from build123d import *

# Parameters (mm, degrees)
SKETCH1_R           = 2.4
BOSS_EXTRUDE1_DEPTH = 2.5
BOSS_EXTRUDE2_DEPTH = 20
BOSS_EXTRUDE3_DEPTH = 40
BOSS_EXTRUDE4_START = -20
BOSS_EXTRUDE4_DEPTH = 20
CUT_EXTRUDE1_DEPTH  = 3


with BuildPart() as part:
    # Sketch1 → Boss-Extrude1 (new body)
    with BuildSketch(Plane.XY):
        with BuildLine():
            ThreePointArc((-21, -11), (-32, 0), (-21, 11))
            Line((-21, 11), (79, 11))
            ThreePointArc((79, 11), (82.762221577, 10.336618829), (86.070663707, 8.426488874))
            Line((86.070663707, 8.426488874), (90.570176974, 13.788799976))
            ThreePointArc((90.570176974, 13.788799976), (85.15636258, 16.914467174), (79, 18))
            Line((79, 18), (-21, 18))
            ThreePointArc((-21, 18), (-39, 0), (-21, -18))
            Line((-21, -18), (63.896206639, -18))
            Line((63.896206639, -18), (69.769904057, -11))
            Line((69.769904057, -11), (-21, -11))
        make_face()
        with Locations((10, -14.5)):
            Circle(SKETCH1_R, mode=Mode.SUBTRACT)
        with Locations((-10, -14.5)):
            Circle(SKETCH1_R, mode=Mode.SUBTRACT)
        with Locations((10, 14.5)):
            Circle(SKETCH1_R, mode=Mode.SUBTRACT)
        with Locations((-10, 14.5)):
            Circle(SKETCH1_R, mode=Mode.SUBTRACT)
    extrude(amount=BOSS_EXTRUDE1_DEPTH)

    # Sketch1<3> → Boss-Extrude2 (add)
    with BuildSketch(Plane.XY):
        with BuildLine():
            ThreePointArc((79, 18), (85.15636258, 16.914467174), (90.570176974, 13.788799976))
            Line((90.570176974, 13.788799976), (93.141327413, 16.852977749))
            ThreePointArc((93.141327413, 16.852977749), (86.524443153, 20.673237657), (79, 22))
            Line((79, 22), (-21, 22))
            ThreePointArc((-21, 22), (-43, 0), (-21, -22))
            Line((-21, -22), (60.539808114, -22))
            Line((60.539808114, -22), (63.896206639, -18))
            Line((63.896206639, -18), (-21, -18))
            ThreePointArc((-21, -18), (-39, 0), (-21, 18))
            Line((-21, 18), (79, 18))
        make_face()
    extrude(amount=BOSS_EXTRUDE2_DEPTH)

    # Sketch1<4> → Boss-Extrude3 (add)
    with BuildSketch(Plane.XY):
        with BuildLine():
            Line((86.070663707, 8.426488874), (79, 0))
            Line((79, 0), (69.769904057, -11))
            Line((69.769904057, -11), (73.686125925, -11))
            Line((73.686125925, -11), (88.100757974, 6.17868953))
            ThreePointArc((88.100757974, 6.17868953), (87.163447205, 7.372796602), (86.070663707, 8.426488874))
        make_face()
        with BuildLine():
            Line((90.570176974, 13.788799976), (86.070663707, 8.426488874))
            ThreePointArc((86.070663707, 8.426488874), (87.163447205, 7.372796602), (88.100757974, 6.17868953))
            Line((88.100757974, 6.17868953), (92.706481677, 11.6675773))
            ThreePointArc((92.706481677, 11.6675773), (91.682754612, 12.772929791), (90.570176974, 13.788799976))
        make_face()
        with BuildLine():
            Line((93.141327413, 16.852977749), (90.570176974, 13.788799976))
            ThreePointArc((90.570176974, 13.788799976), (91.682754612, 12.772929791), (92.706481677, 11.6675773))
            Line((92.706481677, 11.6675773), (95.307364493, 14.76718874))
            ThreePointArc((95.307364493, 14.76718874), (94.260024202, 15.847134168), (93.141327413, 16.852977749))
        make_face()
        with BuildLine():
            Line((117.567256581, 45.962666587), (93.141327413, 16.852977749))
            ThreePointArc((93.141327413, 16.852977749), (94.260024202, 15.847134168), (95.307364493, 14.76718874))
            Line((95.307364493, 14.76718874), (119.865389911, 44.034303758))
            Line((119.865389911, 44.034303758), (117.567256581, 45.962666587))
        make_face()
        Polygon((64.456029982, -22), (60.539808114, -22), (40.432743419, -45.962666587), (42.730876748, -47.891029416), align=None)
        Polygon((67.812428507, -18), (63.896206639, -18), (60.539808114, -22), (64.456029982, -22), align=None)
        Polygon((73.686125925, -11), (69.769904057, -11), (63.896206639, -18), (67.812428507, -18), align=None)
    extrude(amount=BOSS_EXTRUDE3_DEPTH)

    # Sketch1<5> → Boss-Extrude4 (add)
    with BuildSketch(Plane.XY.offset(BOSS_EXTRUDE4_START)):
        Polygon((64.456029982, -22), (60.539808114, -22), (40.432743419, -45.962666587), (42.730876748, -47.891029416), align=None)
        with BuildLine():
            Line((117.567256581, 45.962666587), (93.141327413, 16.852977749))
            ThreePointArc((93.141327413, 16.852977749), (94.260024202, 15.847134168), (95.307364493, 14.76718874))
            Line((95.307364493, 14.76718874), (119.865389911, 44.034303758))
            Line((119.865389911, 44.034303758), (117.567256581, 45.962666587))
        make_face()
        with BuildLine():
            Line((90.570176974, 13.788799976), (86.070663707, 8.426488874))
            ThreePointArc((86.070663707, 8.426488874), (87.163447205, 7.372796602), (88.100757974, 6.17868953))
            Line((88.100757974, 6.17868953), (92.706481677, 11.6675773))
            ThreePointArc((92.706481677, 11.6675773), (91.682754612, 12.772929791), (90.570176974, 13.788799976))
        make_face()
        with BuildLine():
            Line((93.141327413, 16.852977749), (90.570176974, 13.788799976))
            ThreePointArc((90.570176974, 13.788799976), (91.682754612, 12.772929791), (92.706481677, 11.6675773))
            Line((92.706481677, 11.6675773), (95.307364493, 14.76718874))
            ThreePointArc((95.307364493, 14.76718874), (94.260024202, 15.847134168), (93.141327413, 16.852977749))
        make_face()
        with BuildLine():
            Line((86.070663707, 8.426488874), (79, 0))
            Line((79, 0), (69.769904057, -11))
            Line((69.769904057, -11), (73.686125925, -11))
            Line((73.686125925, -11), (88.100757974, 6.17868953))
            ThreePointArc((88.100757974, 6.17868953), (87.163447205, 7.372796602), (86.070663707, 8.426488874))
        make_face()
        Polygon((73.686125925, -11), (69.769904057, -11), (63.896206639, -18), (67.812428507, -18), align=None)
        Polygon((67.812428507, -18), (63.896206639, -18), (60.539808114, -22), (64.456029982, -22), align=None)
    extrude(amount=BOSS_EXTRUDE4_DEPTH)

    # Sketch5 → Cut-Extrude1 (cut)
    with BuildSketch(Plane(origin=(48.657236347, -40.828269073, 0), x_dir=(0, 0, -1), z_dir=(0.7660444431189747, -0.6427876096865435, 0))):
        with BuildLine():
            ThreePointArc((-17.6, -2.819778835), (-20, -0.419778835), (-22.4, -2.819778835))
            Line((-22.4, -2.819778835), (-20, -2.819778835))
            Line((-20, -2.819778835), (-20, -5.219778835))
            ThreePointArc((-20, -5.219778835), (-18.302943725, -4.51683511), (-17.6, -2.819778835))
        make_face()
        with BuildLine():
            Line((-20, -2.819778835), (-22.4, -2.819778835))
            ThreePointArc((-22.4, -2.819778835), (-21.697056275, -4.51683511), (-20, -5.219778835))
            Line((-20, -5.219778835), (-20, -2.819778835))
        make_face()
        with BuildLine():
            Line((0, -5.219778835), (0, -2.819778835))
            Line((0, -2.819778835), (2.4, -2.819778835))
            ThreePointArc((2.4, -2.819778835), (-1.697056275, -1.12272256), (0, -5.219778835))
        make_face()
        with BuildLine():
            Line((2.4, -2.819778835), (0, -2.819778835))
            Line((0, -2.819778835), (0, -5.219778835))
            ThreePointArc((0, -5.219778835), (1.697056275, -4.51683511), (2.4, -2.819778835))
        make_face()
        with BuildLine():
            ThreePointArc((-17.6, 104.380221165), (-18.302943725, 106.07727744), (-20, 106.780221165))
            Line((-20, 106.780221165), (-20, 104.380221165))
            Line((-20, 104.380221165), (-22.4, 104.380221165))
            ThreePointArc((-22.4, 104.380221165), (-20, 101.980221165), (-17.6, 104.380221165))
        make_face()
        with BuildLine():
            Line((-20, 104.380221165), (-20, 106.780221165))
            ThreePointArc((-20, 106.780221165), (-21.697056275, 106.07727744), (-22.4, 104.380221165))
            Line((-22.4, 104.380221165), (-20, 104.380221165))
        make_face()
        with BuildLine():
            ThreePointArc((2.4, 104.380221165), (1.697056275, 106.07727744), (0, 106.780221165))
            Line((0, 106.780221165), (0, 104.380221165))
            Line((0, 104.380221165), (2.4, 104.380221165))
        make_face()
        with BuildLine():
            Line((0, 104.380221165), (0, 106.780221165))
            ThreePointArc((0, 106.780221165), (-1.697056275, 102.68316489), (2.4, 104.380221165))
            Line((2.4, 104.380221165), (0, 104.380221165))
        make_face()
    extrude(amount=-CUT_EXTRUDE1_DEPTH, mode=Mode.SUBTRACT)


solid = part.part
CAD build for the part. Positions are in the model's coordinates, mm. A direction names the side the tool comes from. Give positions to 0.01 mm unless a question says otherwise; leave off trailing zeros. Write each loop counter-clockwise with the first axis right and the second up, starting at its lowest first coordinate (ties: lowest second). Pieces come first, ordered by that corner, then holes. Notation, with made-up numbers: (30.5, -16) - (35.5, -16) arc R23 ccw to (35.5, -1) - close; hole circle Ø9 at (-31.5, 79). An arc over 180 degrees is marked (long way). Answer as CSV lines item,"result".
Q1. Band-saw the part on C-C (z = 13). Give the cut face in (x, y), and give its area (3 significant figures).
Result set:
outline,"(-21, -22) - (60.54, -22) - (40.43, -45.96) - (42.73, -47.89) - (119.87, 44.03) - (117.57, 45.96) - (93.14, 16.85) arc R22 ccw to (79, 22) - (-21, 22) arc R22 ccw to start; hole (-21, -18) - (63.9, -18) - (90.57, 13.79) arc R18 ccw to (79, 18) - (-21, 18) arc R18 ccw to start"
area,"1,400 mm²"
Q2. Pull direction X, two halves, no side cores. Call faces 5 (the face through (30, 22, 10)), 6 (the face through (-43, 0, 10)), 7 (the face through (-32, 0, 1)), 8 (the face through (-10.31, 16.88, 1.23)): released by +X, released by -X, zero draft, split by the parting line, or undercut.
Result set:
face 5,"zero draft"
face 6,"released by -X"
face 7,"undercut"
face 8,"undercut"
Q3. Band-saw the part on A-A (x = -5). Give the cut face in (y, z).
Result set:
outline,"(-22, 0) - (-11, 0) - (-11, 2.5) - (-18, 2.5) - (-18, 20) - (-22, 20) - close; (11, 0) - (22, 0) - (22, 20) - (18, 20) - (18, 2.5) - (11, 2.5) - close"
Q4. Flat gauge pins, fed straight in: pin 1 Ø1 at (y, z) = (-33.5, 9.5) entering from +X; pin 2 Ø6 at (x, z) = (18, 13) entering from +Y; pin 3 Ø4 at (x, y) = (10, 14.5) entering from +Z; pin 4 Ø22 at (x, y) = (11.5, -5) entering from +Z. Where does each tip first touch, or does it go through?
Result set:
pin 1,"x = 55.23"
pin 2,"y = 22"
pin 3,"through"
pin 4,"z = 2.5"
Q5. Band-saw the part on D-D (z = -9.5). Give the cut face in (x, y).
Result set:
outline,"(40.43, -45.96) - (42.73, -47.89) - (119.87, 44.03) - (117.57, 45.96) - close"
Q6. 3-axis set-ups, long thin cutter, end or side, ignore diameter. For faces 1 (the face through (86.625, 20.636, 9.86)), 2 (the face through (19, -22, 10)), 3 (the face through (-39, 0, 11)), 4 (the face through (10, 20, 20)): which of +Z, -Z, +X, -X, +Y, -Y reach the whole face in a straight line?
Result set:
face 1,"+Z, -Z, +Y"
face 2,"+Z, -Z, -X"
face 3,"+Z"
face 4,"+Z, -X, +Y"
Q7. Band-saw the part on B-B (y = -6.5). Give the cut face in (x, z), and give its area (3 significant figures).
Result set:
outline,"(-42.02, 0) - (-29.87, 0) - (-29.87, 2.5) - (-37.79, 2.5) - (-37.79, 20) - (-42.02, 20) - close; (73.55, -20) - (77.46, -20) - (77.46, 40) - (73.55, 40) - close"
area,"339 mm²"
Q8. Drill centre lines: line 1 (Y direction, x = 10, z = 0.65); line 2 (X direction, y = 10, z = -7); line 3 (Z direction, x = 86, y = 17). Where is each one in solid material? Low to high. Write a range as from..to.
Result set:
line 1,"-22..-16.9, -12.1..-11, 11..12.1, 16.9..22"
line 2,"87.39..91.31"
line 3,"0..20"
